Geometry check sheet. Reference: the model listing, model coordinates, mm. A direction names the side the tool comes from. Coordinates: 2 decimals unless noted, no trailing zeros. Loops run counter-clockwise (first coordinate to the right, second up) from the corner with the lowest first, then second, coordinate; pieces in that order, holes last. Notation, with made-up numbers: (29, 77) - (52, 77) arc R19 ccw to (52, 82) - close; hole circle Ø8 at (-18, -10). An arc over 180 degrees is marked (long way). Write item = value, one per line. Start each with the question number.
from build123d import *

# Parameters (mm, degrees)
CUT_EXTRUDE_1_DEPTH = 3
FILLET_1_R          = 0.3
CHAMFER_1_SIZE      = 1


with BuildPart() as part:
    # Эскиз1 → Повернуть1 (revolve)
    with BuildSketch(Plane.XY, mode=Mode.PRIVATE) as revolve_1_sk:
        Polygon((0, 0), (0, 5.9), (0.5, 5.9), (4, 3), (25, 3), (25, 0), align=None)
    revolve(revolve_1_sk.sketch.rotate(Axis((0, 0, 0), (1, 0, 0)), 90), axis=Axis((0, 0, 0), (1, 0, 0)))  # turned: the seam where the file's is

    # Эскиз2 → Вырез-Вытянуть1 (cut)
    with BuildSketch(Plane.ZY):
        Polygon((1.154700538, 2), (-1.154700538, 2), (-2.309401077, 0), (-1.154700538, -2), (1.154700538, -2), (2.309401077, 0), align=None)
    extrude(amount=-CUT_EXTRUDE_1_DEPTH, mode=Mode.SUBTRACT)

    # Скругление1
    fillet_1_edges = [part.edges().sort_by_distance(p)[0] for p in [
        (0, 0, -5.9),
    ]]
    fillet(fillet_1_edges, radius=FILLET_1_R)

    # Фаска1
    chamfer_1_edges = [part.edges().sort_by_distance(p)[0] for p in [
        (25, 0, -3),
    ]]
    chamfer(chamfer_1_edges, length=CHAMFER_1_SIZE)


solid = part.part
(1) Sectioned sample at B-B on x = 10. Enter the section's corners in (y, z), plus the area to 3 significant figures.
(2) Depth check by flat-ended pin: pin 1 (2 mm diameter, centred on y = 0.5, z = -0.5, fed in from -X); pin 2 (6 mm diameter, centred on x = 16, z = -3.5, fed in from -Y); pin 3 (1 mm diameter, centred on y = 1, z = -1.5, fed in from -X); pin 4 (1.2 mm diameter, centred on x = 1, z = -0.5, fed in from +Y). Enter the tip coordinate at first touch or a pass-through.
(3) Scan lines: line 1 (Y direction, x = 23, z = 0); line 2 (X direction, y = -1.5, z = -1); line 3 (Y direction, x = 7.25, z = 0.75). Record each from-to range of solid material in increasing order.
(4) Tool access check on faces 1 (the face through (0, 2.4, 0.1)), 2 (the face through (14.14, -0.9, 2.86)), 3 (the face through (1.48, -0.99, -1.74)). Record the directions out of +Z, -Z, +X, -X, +Y, -Y that give a thin tool (end or side, any length) a straight path to the whole face; none if there is none.
(5) Draft check along Z on faces 4 (the face through (25, 0, 0)), 5 (the face through (1.479, -1.014, 1.724)), 6 (the face through (3.83, -0.943, 2.996)). Enter one of: pulls with the +Z half, pulls with the -Z half, needs draft (parallel to the pull), parting line crosses it, or undercut.
(6) Sectioned sample at A-A on z = 0. Enter the section's corners in (x, y), plus the area to 3 significant figures.
Working result:
q1.outline = circle Ø6 at (0, 0)
q1.area = 28.3 mm2
q2.pin_1 = 3
q2.pin_2 = -2.96
q2.pin_3 = 0
q2.pin_4 = 5.9
q3.line_1 = -3 to 3
q3.line_2 = 3 to 25
q3.line_3 = -2.9 to 2.9
q4.face_1 = +Z, -Z, -X, +Y, -Y
q4.face_2 = +X
q4.face_3 = -X
q5.face_4 = needs draft
q5.face_5 = undercut
q5.face_6 = parting line crosses it
q6.outline = (0, -5.6) arc R0.3 ccw to (0.3, -5.9) - (0.5, -5.9) - (4, -3) - (24, -3) - (25, -2) - (25, 2) - (24, 3) - (4, 3) - (0.5, 5.9) - (0.3, 5.9) arc R0.3 ccw to (0, 5.6) - (0, 2) - (3, 2) - (3, -2) - (0, -2) - close
q6.area = 150 mm2
